Geometry check sheet. Reference: the model listing, model coordinates, mm. Face numbers are marked on the shaded views. A direction names the side the tool comes from. Round coordinates to 2 decimals unless told otherwise and drop trailing zeros. Order: outer loops, then holes, each group sorted by start corner. A loop starts at its lowest first (then second) coordinate and runs counter-clockwise, first axis right, second up. Notation, with made-up numbers: (23, -10.5) - (69, -10.5) arc R16 ccw to (69, 4.5) - close; hole circle Ø7 at (-8, -32.75). An arc over 180 degrees is marked (long way). Return JSON: item names as keys, results as strings. Group by question number.
Q1. Sectioned sample at B-B, the plane x = 47. Record the cut outline in (y, z).
Q2. Material ranges on line 1 along Y through (x, z) = (30, 28.35); line 2 along Z through (x, y) = (32, 0); line 3 along Z through (x, y) = (21, 0), recorded low to high.
Q3. Tool access check on the marked faces 4, 5, 6, 7 and 8. Record the directions out of +Z, -Z, +X, -X, +Y, -Y that give a thin tool (end or side, any length) a straight path to the whole face; none if there is none.
Q4. Sectioned sample at A-A, the plane x = 43. Record the cut outline in (y, z), then the cut area to 3 significant figures.
Q5. Gauge pin test, flat ends, axial feed: pin 1 Ø4 at (x, y) = (39, 5) entering from +Z; pin 2 Ø2 at (x, z) = (50, 27) entering from +Y; pin 3 Ø2 at (x, z) = (43.5, 27) entering from -Y. Record the tip position at first contact, or that the pin passes through.
Q6. Draft check along Z on the marked faces 1, 2 and 3. Enter one of: pulls with the +Z half, pulls with the -Z half, needs draft (parallel to the pull), parting line crosses it, or undercut.
```python
from build123d import *

# Parameters (mm, degrees)
PAD023_DEPTH         = 34
POCKET032_DEPTH      = 6.864961
POCKET032_DEPTH_BACK = 6.864961
POCKET033_DEPTH      = 3.5
SKETCH057_R          = 2.15
POCKET034_DEPTH      = 21
POCKET035_DEPTH      = 3.5
SKETCH069_R          = 3.15
POCKET036_DEPTH      = 4


with BuildPart() as part:
    # Sketch054 → Pad023 (new body)
    with BuildSketch(Plane(origin=(20, 0, 28.35), x_dir=(0, -1, 0), z_dir=(-1, 0, 0))):
        with BuildLine():
            Line((-0.353553, 6.717514), (-6.717514, 0.353553))
            ThreePointArc((-6.717514, 0.353553), (-6.863961, 0), (-6.717514, -0.353553))
            Line((-0.353553, -6.717514), (-6.717514, -0.353553))
            ThreePointArc((-0.353553, -6.717514), (0, -6.863961), (0.353553, -6.717514))
            Line((6.717514, -0.353553), (0.353553, -6.717514))
            ThreePointArc((6.717514, -0.353553), (6.863961, 0), (6.717514, 0.353553))
            Line((0.353553, 6.717514), (6.717514, 0.353553))
            ThreePointArc((0.353553, 6.717514), (0, 6.863961), (-0.353553, 6.717514))
        make_face()
    extrude(amount=-PAD023_DEPTH)

    # Sketch067 → Pocket032 (cut, two sides)
    with BuildSketch(Plane(origin=(47, 0, 28.35), x_dir=(1, 0, 0), z_dir=(0, -1, 0))) as pocket032_sk:
        Polygon((-10.885376, 12.57942), (24.170823, 12.57942), (24.170823, 4.191882), (-3.027771, 4.191882), align=None)
        Polygon((24.170823, -4.191882), (-3.027771, -4.191882), (-11.580444, -12.57942), (24.170823, -12.57942), align=None)
    extrude(amount=-POCKET032_DEPTH, mode=Mode.SUBTRACT)
    extrude(pocket032_sk.sketch, amount=POCKET032_DEPTH_BACK, mode=Mode.SUBTRACT)

    # Sketch056 → Pocket033 (cut, symmetric)
    with BuildSketch(Plane(origin=(47, 0, 28.35), x_dir=(1, 0, 0), z_dir=(0, -1, 0))):
        with BuildLine():
            Line((20.145038, 2), (1.859623, 6.916416))
            ThreePointArc((1.859623, 6.916416), (-7.162053, 0), (1.859623, -6.916416))
            Line((20.145038, -2), (1.859623, -6.916416))
            Line((20.145038, 2), (20.145038, -2))
        make_face()
        with BuildLine():
            ThreePointArc((0.844932, 3.142521), (-3.254128, 0), (0.844932, -3.142521))
            Line((0.844932, -3.142521), (12.532776, 0))
            Line((0.844932, 3.142521), (12.532776, 0))
        make_face(mode=Mode.SUBTRACT)
    extrude(amount=POCKET033_DEPTH, both=True, mode=Mode.SUBTRACT)

    # Sketch057 → Pocket034 (cut)
    with BuildSketch(Plane(origin=(20, 0, 28.35), x_dir=(0, -1, 0), z_dir=(-1, 0, 0))):
        Circle(SKETCH057_R)
    extrude(amount=-POCKET034_DEPTH, mode=Mode.SUBTRACT)

    # Sketch068 → Pocket035 (cut)
    with BuildSketch(Plane(origin=(23, 0, 28.35), x_dir=(0, -0.707107, 0.707107), z_dir=(-1, 0, 0))):
        Polygon((-3.65, -3.65), (3.65, -3.65), (3.65, 3.65), (4.4, 8.65), (-4.4, 8.65), (-3.65, 3.65), align=None)
    extrude(amount=-POCKET035_DEPTH, mode=Mode.SUBTRACT)

    # Sketch069 → Pocket036 (cut)
    with BuildSketch(Plane(origin=(20, 0, 28.35), x_dir=(0, -1, 0), z_dir=(-1, 0, 0))):
        Circle(SKETCH069_R)
    extrude(amount=-POCKET036_DEPTH, mode=Mode.SUBTRACT)


solid = part.part
```
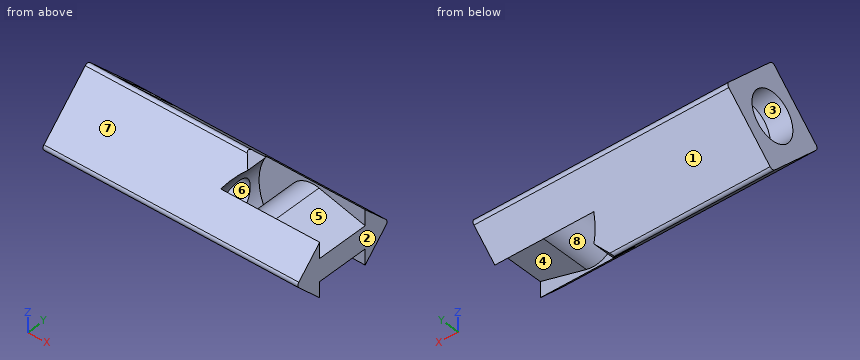
Reply:
{
 "1": {"outline": "(-6.72, 28) - (-3.5, 24.78) - (-3.5, 25.1) - (3.5, 25.1) - (3.5, 24.78) - (6.72, 28) arc R0.5 ccw to (6.72, 28.7) - (3.5, 31.92) - (3.5, 31.6) - (-3.5, 31.6) - (-3.5, 31.92) - (-6.72, 28.7) arc R0.5 ccw to start"},
 "2": {"line 1": "-6.86 to -2.15, 2.15 to 6.86", "line 2": "21.49 to 26.2, 30.5 to 35.21", "line 3": "21.49 to 25.2, 31.5 to 35.21"},
 "3": {"face 4": "-Z, +X", "face 5": "+Z, +X", "face 6": "-X", "face 7": "+Z, +X, -X, -Y", "face 8": "none"},
 "4": {"outline": "(-6.72, 28) - (-3.5, 24.78) - (-3.5, 31.92) - (-6.72, 28.7) arc R0.5 ccw to start; (3.5, 24.78) - (6.72, 28) arc R0.5 ccw to (6.72, 28.7) - (3.5, 31.92) - close", "area": "25.4 mm^2"},
 "5": {"pin 1": "z = 32.42", "pin 2": "y = 6.72", "pin 3": "y = -6.72"},
 "6": {"face 1": "pulls with the -Z half", "face 2": "needs draft", "face 3": "undercut"}
}
